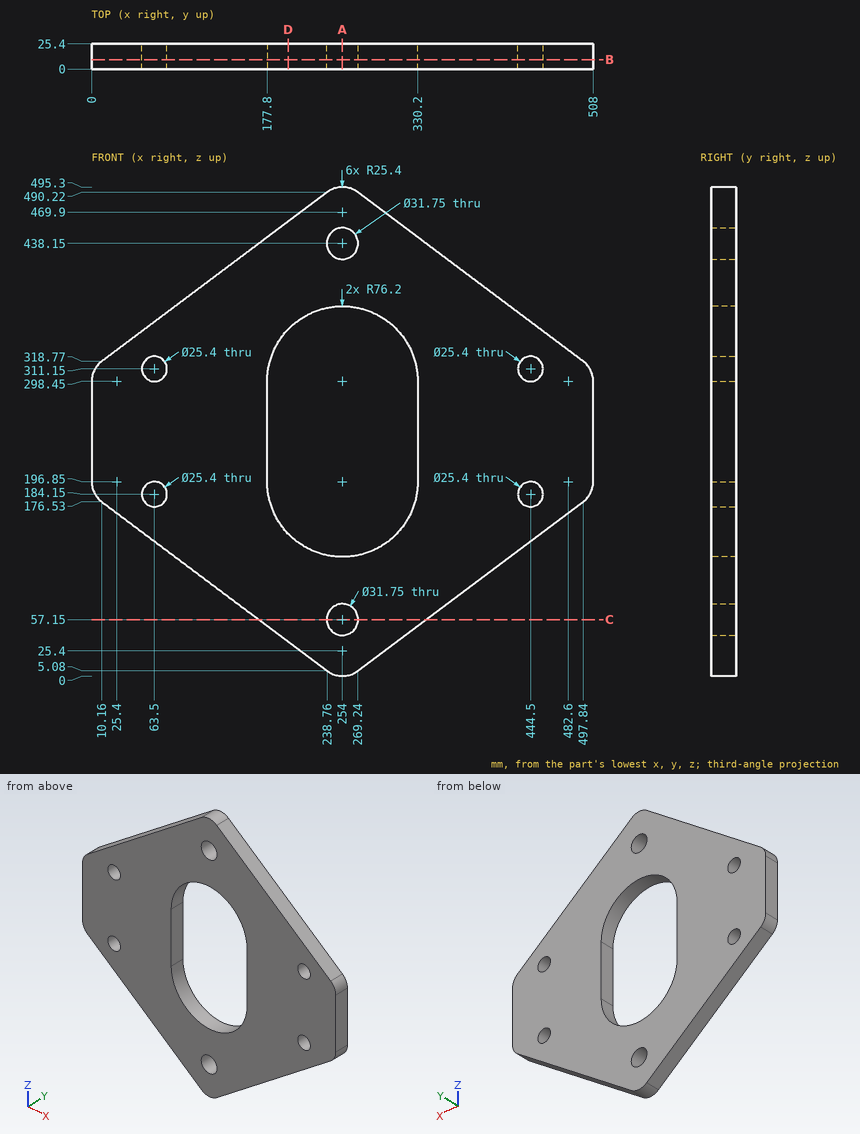
Part print with two shaded views. Sizes in mm from the minimum x, y, z corner. Round coordinates to 2 decimals unless told otherwise and drop trailing zeros. Order: outer loops, then holes, each group sorted by start corner. A loop starts at its lowest first (then second) coordinate and runs counter-clockwise, first axis right, second up. Notation, with made-up numbers: M 88,-37.5 L 101,-37.5 A24 ccw 101,-5.5 Z; hole C 78.25,7.25 d5. An arc over 180 degrees is marked long. Put each result on its own line as item: value. Start each with the question number.
1. Slice it at A-A on x = 254. List the corners of the cut face in (y, z) (3 decimals), then the cut area to 3 significant figures.
2. Drill centre lines: probe 1 along Z at (x, y) = (254, 12) (3 decimals); probe 2 along Z at (x, y) = (63.5, 12) (3 decimals); probe 3 along X at (y, z) = (19, 237). Where is each one in solid material? Low to high. Write a range as [from, to].
3. Slice it at D-D on x = 199. List the corners of the cut face in (y, z), then the cut area to 3 significant figures.
4. Slice it at B-B on y = 9.5. List the corners of the cut face in (x, z) (3 decimals), then the cut area to 3 significant figures.
5. Slice it at C-C on z = 57.15. List the corners of the cut face in (x, y) (3 decimals), then the cut area to 3 significant figures.
6. Drop flat-ended pins along their axis: pin 1 (1.5 mm diameter, centred on x = 355.5, y = 18.5, fed in from +Z); pin 2 (6 mm diameter, centred on x = 454.5, y = 21, fed in from +Z) (3 decimals); pin 3 (12 mm diameter, centred on y = 14, z = 171, fed in from +X). Give the stop position or say it passes through.
Findings:
1. outline: M 0,0 L 25.4,0 L 25.4,41.275 L 0,41.275 Z; M 0,73.025 L 25.4,73.025 L 25.4,120.65 L 0,120.65 Z; M 0,374.65 L 25.4,374.65 L 25.4,422.275 L 0,422.275 Z; M 0,454.025 L 25.4,454.025 L 25.4,495.3 L 0,495.3 Z
1. area: 4,520 mm2
2. probe 1: [0, 41.275], [73.025, 120.65], [374.65, 422.275], [454.025, 495.3]
2. probe 2: [136.525, 171.45], [196.85, 298.45], [323.85, 358.775]
2. probe 3: [0, 177.8], [330.2, 508]
3. outline: M 0,34.9 L 25.4,34.9 L 25.4,144.11 L 0,144.11 Z; M 0,351.19 L 25.4,351.19 L 25.4,460.4 L 0,460.4 Z
3. area: 5,550 mm2
4. outline: M 0,196.85 A25.4 ccw 10.16,176.53 L 238.76,5.08 A25.4 ccw 269.24,5.08 L 497.84,176.53 A25.4 ccw 508,196.85 L 508,298.45 A25.4 ccw 497.84,318.77 L 269.24,490.22 A25.4 ccw 238.76,490.22 L 10.16,318.77 A25.4 ccw 0,298.45 Z; hole C 63.5,184.15 d25.4; hole C 63.5,311.15 d25.4; hole M 177.8,196.85 A76.2 ccw 330.2,196.85 L 330.2,298.45 A76.2 ccw 177.8,298.45 Z; hole C 254,57.15 d31.75; hole C 254,438.15 d31.75; hole C 444.5,184.15 d25.4; hole C 444.5,311.15 d25.4
4. area: 124,000 mm2
5. outline: M 169.333,0 L 238.125,0 L 238.125,25.4 L 169.333,25.4 Z; M 269.875,0 L 338.667,0 L 338.667,25.4 L 269.875,25.4 Z
5. area: 3,490 mm2
6. pin 1: z = 426.09
6. pin 2: z = 353.525
6. pin 3: x = 498.45
